Here's how the part is built. I have some questions about the finished solid (model axes, mm). A direction names the side the tool comes from. Round coordinates to 2 decimals unless told otherwise and drop trailing zeros. Loops run counter-clockwise (first coordinate to the right, second up) from the corner with the lowest first, then second, coordinate; pieces in that order, holes last. Notation, with made-up numbers: M 35,28.25 L 52,28.25 A9 cw 52,32.25 Z; hole C 75.25,-15 d2. An arc over 180 degrees is marked long. Answer as a JSON object with one key per item and string values.
from build123d import *

# Parameters (mm, degrees)
BOSS_EXTRUDE1_DEPTH = 8
BOSS_EXTRUDE2_DEPTH = 30


with BuildPart() as part:
    # Sketch1 → Boss-Extrude1 (new body)
    with BuildSketch(Plane.XY):
        Polygon((2.441453407, 4.443445202), (-2.627409721, 4.336083274), (-5.068863129, -0.107361928), (-2.441453407, -4.443445202), (2.627409721, -4.336083274), (5.068863129, 0.107361928), align=None)
        with BuildLine():
            Line((1.75, 2.004770405), (1.75, -1.975229595))
            ThreePointArc((1.75, -1.975229595), (0, -2.638945235), (-1.75, -1.975229595))
            Line((-1.75, -1.975229595), (-1.75, 2.004770405))
            ThreePointArc((-1.75, 2.004770405), (0, 2.661128403), (1.75, 2.004770405))
        make_face(mode=Mode.SUBTRACT)
    extrude(amount=BOSS_EXTRUDE1_DEPTH)

    # Sketch2 → Boss-Extrude2 (add)
    with BuildSketch(Plane(origin=(0, 0, 0), x_dir=(-1, 0, 0), z_dir=(0, 0, -1))):
        Polygon((2.627409721, 4.336083274), (-2.441453407, 4.443445202), (-5.068863129, 0.107361928), (-2.627409721, -4.336083274), (2.441453407, -4.443445202), (5.068863129, -0.107361928), align=None)
    extrude(amount=BOSS_EXTRUDE2_DEPTH)


solid = part.part
Item 1: I want a section at A-A, the plane z = 4. Please give me the cut outline in (x, y).
Resolved:
{"outline": "M -5.07,-0.11 L -2.44,-4.44 L 2.63,-4.34 L 5.07,0.11 L 2.44,4.44 L -2.63,4.34 Z; hole M -1.75,-1.98 A2.64 ccw 1.75,-1.98 L 1.75,2 A2.66 ccw -1.75,2 Z"}
Item 2: On a 3-axis mill with a long thin cutter (end or side, diameter ignored), from which of +Z, -Z, +X, -X, +Y, -Y can I reach the whole of each face in a straight line? I mean faces 1 (the face through (3.737, 2.306, -10.734)), 2 (the face through (0, 0, 0)). Say none if no direction works.
Resolved:
{"face 1": "+Z, -Z, +X, +Y", "face 2": "+Z"}
Item 3: I want a section at B-B, the plane y = -1.5. Please give me the cut outline in (x, z) (3 decimals).
Resolved:
{"outline": "M -4.225,-30 L 4.186,-30 L 4.186,8 L 1.75,8 L 1.75,0 L -1.75,0 L -1.75,8 L -4.225,8 Z"}
Item 4: Please list where these lines run through material, in increasing order: probe 1 along Z at (x, y) = (0.25, 0.75); probe 2 along X at (y, z) = (-2.25, 4.5); probe 3 along Y at (x, z) = (2.25, 2). Write a range as from..to.
Resolved:
{"probe 1": "-30..0", "probe 2": "-3.77..-1.38, 1.38..3.77", "probe 3": "-4.34..4.44"}
Item 5: I want a section at D-D, the plane x = -1. Please give me the cut outline in (y, z), then the cut area to 3 significant figures.
Resolved:
{"outline": "M -4.41,-30 L 4.37,-30 L 4.37,8 L 2.47,8 L 2.47,0 L -2.44,0 L -2.44,8 L -4.41,8 Z", "area": "295 mm²"}
Item 6: If we mould it in two halves opening along Y, with no side actions, what happens to faces 3 (the face through (2, 0, 8)), 4 (the face through (1.75, 0, 4)), 5 (the face through (-3.865, 2.083, -10.734)), 6 (the face through (-3.737, -2.306, -10.734))? For each: pulls with the +Y half, pulls with the -Y half, needs draft (parallel to the pull), parting line crosses it, or undercut.
Resolved:
{"face 3": "needs draft", "face 4": "undercut", "face 5": "pulls with the +Y half", "face 6": "pulls with the -Y half"}
Item 7: I'm going to push flat-ended pins straight in: pin 1 Ø1 at (y, z) = (-2.5, -19.5) entering from +X; pin 2 Ø3 at (y, z) = (0, 3) entering from +X; pin 3 Ø1 at (x, y) = (0, 0.5) entering from +Z; pin 4 Ø1 at (x, z) = (-2, -9.5) entering from +Y. Where does each tip first touch, or does it pass through?
Resolved:
{"pin 1": "x = 3.91", "pin 2": "x = 5.07", "pin 3": "z = 0", "pin 4": "y = 4.36"}
Item 8: I want a section at C-C, the plane z = -18. Please give me the cut outline in (x, y).
Resolved:
{"outline": "M -5.07,-0.11 L -2.44,-4.44 L 2.63,-4.34 L 5.07,0.11 L 2.44,4.44 L -2.63,4.34 Z"}
